The listing builds one solid part. Answer for the finished solid, in the listing's coordinates (mm). Round coordinates to 2 decimals unless told otherwise and drop trailing zeros. Write item = value, one per line. Start each with the question number.
1) Straight lines are drawn through the part: line 1 along Z through (x, y) = (-99.5, 6.5); line 2 along Z through (x, y) = (11.5, 8.25); line 3 along Z through (x, y) = (122.5, 0.75). For each, find the intervals that lie inside material, in ascending order.
2) For a pull along Z with two mould halves and no side action, classify faces 1 (the flat face through (111.2, 4.9, 67.2)), 2 (the cylindrical face through (-0.16, 5.07, -57.5)) as released by +Z, released by -Z, zero draft, split by the parting line, or undercut.
3) Given pin 1 Ø6 at (x, y) = (118, 5.5) entering from +Z; pin 2 Ø5 at (y, z) = (8.5, 29) entering from -X; pin 3 Ø5 at (y, z) = (2.5, -104.5) entering from -X, each flat-ended and moving along its own axis, determine where each tip first touches the part or whether it passes through.
4) Section A-A, the plane y = 8.25 is taken. Give the number of separate pieces and of enclosed holes in the cut face, and give its area (3 significant figures).
from build123d import *

# Parameters (mm, degrees)
BOSS_EXTRUDE1_DEPTH = 10
SKETCH2_R           = 3.05
CUT_EXTRUDE1_DEPTH  = 344.838624939
FILLET1_R           = 25
SKETCH3_R           = 4
CUT_EXTRUDE2_DEPTH  = 313.983999349
SKETCH4_R           = 4.05
SKETCH4_W           = 40
SKETCH4_H           = 10
CUT_EXTRUDE3_DEPTH  = 313.983999349
CIRPATTERN1_COUNT   = 3
SKETCH7_R           = 2.05
SKETCH7_R_2         = 1.55
CUT_EXTRUDE4_DEPTH  = 313.983999349
SKETCH8_R           = 42.5
CUT_EXTRUDE5_DEPTH  = 313.983999349


with BuildPart() as part:
    # Sketch1 → Boss-Extrude1 (new body)
    with BuildSketch(Plane(origin=(0, 0, 0), x_dir=(1, 0, 0), z_dir=(0, 1, 0))):
        Polygon((0, -259.807621135), (225, 129.903810568), (-225, 129.903810568), align=None)
    extrude(amount=BOSS_EXTRUDE1_DEPTH)

    # Sketch2 → Cut-Extrude1 (cut, through all)
    with BuildSketch(Plane(origin=(0, 10, 0), x_dir=(1, 0, 0), z_dir=(0, 1, 0))):
        with Locations(Location((-52.5, 60, 0), (0, 0, 270))):
            Circle(SKETCH2_R)
        with Locations(Location((-52.5, -60, 0), (0, 0, 270))):
            Circle(SKETCH2_R)
        with Locations(Location((-52.5, -20, 0), (0, 0, 270))):
            Circle(SKETCH2_R)
        with Locations(Location((-52.5, 20, 0), (0, 0, 270))):
            Circle(SKETCH2_R)
    cut_extrude1 = extrude(amount=-CUT_EXTRUDE1_DEPTH, mode=Mode.SUBTRACT)

    # Mirror1: Cut-Extrude1 across plane
    add(cut_extrude1.mirror(Plane(origin=(0, 0, 0), x_dir=(0, 0, 1), z_dir=(1, 0, 0))), mode=Mode.SUBTRACT)

    # Fillet1
    fillet1_edges = [part.edges().sort_by_distance(p)[0] for p in [
        (-225, 5, -129.903810568),
        (225, 5, -129.903810568),
        (0, 5, 259.807621135),
    ]]
    fillet(fillet1_edges, radius=FILLET1_R)

    # Sketch3 → Cut-Extrude2 (cut, through all)
    with BuildSketch(Plane(origin=(0, 10, 0), x_dir=(1, 0, 0), z_dir=(0, 1, 0))):
        with Locations(Location((0, -209.807621135, 0), (0, 0, 270))):
            Circle(SKETCH3_R)
        with Locations(Location((181.698729811, 104.903810568, 0), (0, 0, 270))):
            Circle(SKETCH3_R)
        with Locations(Location((-181.698729811, 104.903810568, 0), (0, 0, 270))):
            Circle(SKETCH3_R)
    extrude(amount=-CUT_EXTRUDE2_DEPTH, mode=Mode.SUBTRACT)

    # Sketch4 → Cut-Extrude3 (cut, through all)
    with BuildSketch(Plane(origin=(0, 10, 0), x_dir=(1, 0, 0), z_dir=(0, 1, 0))):
        with Locations(Location((0, 104.903810568, 0), (0, 0, 270))):
            Circle(SKETCH4_R)
        with Locations(Location((70, 104.903810568, 0), (0, 0, 270))):
            Circle(SKETCH4_R)
        with Locations(Location((140, 104.903810568, 0), (0, 0, 270))):
            Circle(SKETCH4_R)
        with Locations(Location((-140, 104.903810568, 0), (0, 0, 270))):
            Circle(SKETCH4_R)
        with Locations(Location((-70, 104.903810568, 0), (0, 0, 270))):
            Circle(SKETCH4_R)
        with Locations((35, 104.903810568)):
            Rectangle(SKETCH4_W, SKETCH4_H)
        with Locations((-35, 104.903810568)):
            Rectangle(SKETCH4_W, SKETCH4_H)
        with Locations((-105, 104.903810568)):
            Rectangle(SKETCH4_W, SKETCH4_H)
        with Locations((105, 104.903810568)):
            Rectangle(SKETCH4_W, SKETCH4_H)
    cut_extrude3 = extrude(amount=-CUT_EXTRUDE3_DEPTH, mode=Mode.SUBTRACT)

    # CirPattern1: Cut-Extrude3 ×3 about axis
    cirpattern1_axis = Axis((0, 0, 0), (0, 1, 0))
    for i in range(1, CIRPATTERN1_COUNT):
        add(cut_extrude3.rotate(cirpattern1_axis, i * 360 / CIRPATTERN1_COUNT), mode=Mode.SUBTRACT)

    # Sketch7 → Cut-Extrude4 (cut, through all)
    with BuildSketch(Plane(origin=(0, 10, 0), x_dir=(1, 0, 0), z_dir=(0, 1, 0))):
        with Locations(Location((-12.5, -120, 0), (0, 0, 270))):
            Circle(SKETCH7_R)
        with Locations(Location((12.5, -120, 0), (0, 0, 270))):
            Circle(SKETCH7_R)
        with Locations(Location((-12.557368355, -112.75, 0), (0, 0, 270))):
            Circle(SKETCH7_R_2)
        with Locations(Location((0, -134.5, 0), (0, 0, 270))):
            Circle(SKETCH7_R_2)
        with Locations(Location((12.557368355, -112.75, 0), (0, 0, 270))):
            Circle(SKETCH7_R_2)
    extrude(amount=-CUT_EXTRUDE4_DEPTH, mode=Mode.SUBTRACT)

    # Sketch8 → Cut-Extrude5 (cut, through all)
    with BuildSketch(Plane(origin=(0, 10, 0), x_dir=(1, 0, 0), z_dir=(0, 1, 0))):
        Circle(SKETCH8_R)
        with BuildLine():
            Line((-7.5, 35), (-7.5, 50))
            ThreePointArc((-7.5, 50), (0, 57.5), (7.5, 50))
            Line((7.5, 50), (7.5, 35))
            ThreePointArc((7.5, 35), (0, 27.5), (-7.5, 35))
        make_face()
    extrude(amount=-CUT_EXTRUDE5_DEPTH, mode=Mode.SUBTRACT)


solid = part.part
Geometry check:
q1.line_1 = -129.9 to -109.9, -99.9 to 27.47, 40.13 to 87.47
q1.line_2 = -129.9 to -40.91, 40.91 to 111.62, 113.88 to 118.21, 121.79 to 232.01
q1.line_3 = -129.9 to -109.9, -99.9 to -10.45, -5.89 to 7.22, 7.63 to 47.63
q2.face_1 = released by +Z
q2.face_2 = undercut
q3.pin_1 = 60.62
q3.pin_2 = -134.7
q3.pin_3 = -206.7
q4.separate_pieces = 1
q4.enclosed_holes = 44
q4.area = 74,500 mm2
